from build123d import *

# Parameters (mm, degrees)
EXTRUDE_1_DEPTH          = 6
SKETCH_2_R               = 1.7
CUT_EXTRUDE_1_DEPTH      = 13.806248475
CUT_EXTRUDE_2_DEPTH      = 11.770329614
CUT_EXTRUDE_2_DEPTH_BACK = 11.770329614
SKETCH_3_R               = 1.65
CUT_EXTRUDE_3_REACH      = 14.806


with BuildPart() as part:
    # 草图1 → 凸台-拉伸1 (new body)
    with BuildSketch(Plane.XY):
        with BuildLine():
            Line((-3.5, -7), (3.5, -7))
            ThreePointArc((3.5, -7), (3.853553391, -6.853553391), (4, -6.5))
            Line((4, -6.5), (4, 0.714692101))
            ThreePointArc((4, 0.714692101), (3.991879765, 0.999536647), (3.967545434, 1.28345599))
            Line((3.967545434, 1.28345599), (3.3, 7.113752778))
            ThreePointArc((3.3, 7.113752778), (2.972166218, 7.746241508), (2.306490913, 8))
            Line((2.306490913, 8), (0.3, 8))
            Line((0.3, 8), (0.3, 1.673320053))
            ThreePointArc((0.3, 1.673320053), (0, -1.7), (-0.3, 1.673320053))
            Line((-0.3, 1.673320053), (-0.3, 8))
            Line((-0.3, 8), (-2.306490913, 8))
            ThreePointArc((-2.306490913, 8), (-2.972166218, 7.746241508), (-3.3, 7.113752778))
            Line((-3.3, 7.113752778), (-3.967545434, 1.28345599))
            ThreePointArc((-3.967545434, 1.28345599), (-3.991879765, 0.999536647), (-4, 0.714692101))
            Line((-4, 0.714692101), (-4, -6.5))
            ThreePointArc((-4, -6.5), (-3.853553391, -6.853553391), (-3.5, -7))
        make_face()
    extrude(amount=EXTRUDE_1_DEPTH)

    # 草图2 → 切除-拉伸1 (cut, through all)
    with BuildSketch(Plane(origin=(4, 0, 0), x_dir=(0, 0, -1), z_dir=(1, 0, 0))):
        with Locations((-3, -3.6)):
            Circle(SKETCH_2_R)
    extrude(amount=-CUT_EXTRUDE_1_DEPTH, mode=Mode.SUBTRACT)

    # 草图3 → 切除-拉伸2 (cut, two sides: drawn at the far end of the back side and taken through both)
    with BuildSketch(Plane(origin=(0, 0, 0), x_dir=(0, 0, -1), z_dir=(1, 0, 0)).offset(-CUT_EXTRUDE_2_DEPTH_BACK)):
        with Locations(Location((-3, 4.8, 0), (0, 0, 90))):
            Circle(SKETCH_3_R)
    extrude(amount=CUT_EXTRUDE_2_DEPTH + CUT_EXTRUDE_2_DEPTH_BACK, mode=Mode.SUBTRACT)

    # 草图4 → 切除-拉伸3 (cut, up to next)
    with BuildSketch(Plane.ZY.offset(4), mode=Mode.PRIVATE) as cut_extrude_3_sk1:
        with BuildLine():
            Line((0, -3.172768856), (0, -9.012994764))
            Line((0, -9.012994764), (5.999117319, -9.012994764))
            Line((5.999117319, -9.012994764), (6.094166497, -9.012994764))
            Line((6.094166497, -9.012994764), (6.094166497, -3.1))
            Line((6.094166497, -3.1), (5.999117319, -3.1))
            ThreePointArc((5.999117319, -3.1), (3.035504424, -6.099779322), (0, -3.172768856))
        make_face()
    cut_extrude_3_tool1 = extrude(cut_extrude_3_sk1.sketch, amount=-CUT_EXTRUDE_3_REACH, mode=Mode.PRIVATE) & part.part
    add(cut_extrude_3_tool1.solids().sort_by_distance((-4, -7.143206, 3.078044))[0], mode=Mode.SUBTRACT)


solid = part.part
Part model, mm, in its own coordinate system. A direction names the side the tool comes from. Round coordinates to 2 decimals unless told otherwise and drop trailing zeros. Write each loop counter-clockwise with the first axis right and the second up, starting at its lowest first coordinate (ties: lowest second). Pieces come first, ordered by that corner, then holes. Notation, with made-up numbers: M 79,-38 L 132,-38 A17 cw 132,-15 Z; hole C 60,-25.5 d11. An arc over 180 degrees is marked long. Return JSON: item names as keys, results as strings. Group by question number.
(1) Saw through at C-C on z = 3.65. Write the cut outline in (x, y).
(2) Saw through at B-B on x = -1. Count the separate pieces of the cut face and the enclosed holes in it, then the cut area to 3 significant figures.
(3) Pin check, flat tips, straight feed: pin 1 Ø2 at (x, y) = (2, 2.5) entering from -Z; pin 2 Ø3 at (y, z) = (3.5, 3) entering from -X; pin 3 Ø1.8 at (y, z) = (6, 4) entering from +X. Stop position of each tip, or through.
(4) Drill centre lines: probe 1 along Y at (x, z) = (-1.95, 3); probe 2 along Y at (x, z) = (0.5, 2.55); probe 3 along Y at (x, z) = (1.75, 2). Where is each one in solid material? Low to high.
(5) Two-plate mould, pull along Z, no slides. Class faces 3 (the face through (1, 8, 3)), 4 (the face through (-2.06, 3.15, 3.07)), 5 (the face through (1, 3, 6)): +Z half, -Z half, draft (parallel to the pull), parting line (faces both ways), or undercut.
(6) Saw through at A-A on y = -1.5. Write the cut outline in (x, z), then the cut area to 3 significant figures.
(7) Which spindle directions (+Z, -Z, +X, -X, +Y, -Y) get a long thin tool onto all of the face, cutting with end or side? Do faces 1 (the face through (0.3, 3, 2)), 2 (the face through (3.787, 2.862, 2.958)). Say none if no direction does.
Returned:
{
 "1": {"outline": "M -4,-6.03 L 4,-6.03 L 4,-5.17 L -4,-5.17 Z; M -4,-2.03 L 4,-2.03 L 4,0.71 A5 ccw 3.97,1.28 L 3.74,3.28 L 0.3,3.28 L 0.3,1.67 A1.7 cw long -0.3,1.67 L -0.3,3.28 L -3.74,3.28 L -3.97,1.28 A5 ccw -4,0.71 Z; M -3.39,6.32 L -0.3,6.32 L -0.3,8 L -2.31,8 A1 ccw -3.3,7.11 Z; M 0.3,6.32 L 3.39,6.32 L 3.3,7.11 A1 ccw 2.31,8 L 0.3,8 Z"},
 "2": {"separate pieces": "2", "enclosed holes": "2", "area": "46.6 mm²"},
 "3": {"pin 1": "z = 0", "pin 2": "x = -3.89", "pin 3": "x = 3.51"},
 "4": {"probe 1": "-6.1 to -5.3, -1.9 to 3.15, 6.45 to 8", "probe 2": "-6.07 to -5.24, -1.96 to -1.62, 1.62 to 3.21, 6.39 to 8", "probe 3": "-5.93 to -4.97, -2.23 to 3.49, 6.11 to 8"},
 "5": {"face 3": "draft", "face 4": "undercut", "face 5": "+Z half"},
 "6": {"outline": "M -4,0 L -0.8,0 L -0.8,6 L -4,6 Z; M 0.8,0 L 4,0 L 4,6 L 0.8,6 Z", "area": "38.4 mm²"},
 "7": {"face 1": "+Z, -Z, +Y", "face 2": "+Z, -Z, +X, +Y"}
}
